```python
from build123d import *

# Parameters (mm, degrees)
SKETCH3_R          = 2.15
CUT_EXTRUDE1_DEPTH = 10
CHAMFER1_SIZE      = 0.4
CHAMFER2_SIZE      = 2
CHAMFER3_SIZE      = 2


with BuildPart() as part:
    # Sketch1 → Loft1 section 0
    with BuildSketch(Plane.XY):
        with BuildLine():
            Line((0, 0), (54, 0))
            Line((54, 0), (54, 10))
            Line((54, 10), (0, 10))
            Line((0, 10), (0, 0))
        make_face()
    # Sketch2 → Loft1 section 1
    with BuildSketch(Plane.XY.offset(9)):
        with BuildLine():
            Line((0, 9.5), (54, 9.5))
            Line((54, 9.5), (54, 0.5))
            Line((54, 0.5), (0, 0.5))
            Line((0, 0.5), (0, 9.5))
        make_face()
    loft()

    # Sketch3 → Cut-Extrude1 (cut)
    with BuildSketch(Plane(origin=(0, 0, 0), x_dir=(-1, 0, 0), z_dir=(0, 0, -1))):
        with Locations((-49.5, 5)):
            Circle(SKETCH3_R)
        with Locations((-4.5, 5)):
            Circle(SKETCH3_R)
    extrude(amount=-CUT_EXTRUDE1_DEPTH, mode=Mode.SUBTRACT)

    # Chamfer1
    chamfer1_edges = [part.edges().sort_by_distance(p)[0] for p in [
        (51.65, 5, 9),
        (51.65, 5, 0),
        (6.65, 5, 9),
        (6.65, 5, 0),
    ]]
    chamfer(chamfer1_edges, length=CHAMFER1_SIZE)

    # Chamfer2
    chamfer2_edges = [part.edges().sort_by_distance(p)[0] for p in [
        (0, 9.75, 4.5),
        (54, 9.75, 4.5),
    ]]
    chamfer(chamfer2_edges, length=CHAMFER2_SIZE)

    # Chamfer3
    chamfer3_edges = [part.edges().sort_by_distance(p)[0] for p in [
        (54, 0.25, 4.5),
        (0, 0.25, 4.5),
    ]]
    chamfer(chamfer3_edges, length=CHAMFER3_SIZE)


solid = part.part
```
The listing builds one solid part. Answer for the finished solid, in the listing's coordinates (mm). Give positions to 0.01 mm unless a question says otherwise; leave off trailing zeros. Loops run counter-clockwise (first coordinate to the right, second up) from the corner with the lowest first, then second, coordinate; pieces in that order, holes last. Notation, with made-up numbers: M 22,-20.75 L 69,-20.75 A38 ccw 69,18.25 Z; hole C 36,27 d9. An arc over 180 degrees is marked long. One line per item, written item: value.
Q1. A cutting plane is placed at C-C on x = 36. Determine the outline of the cut face in (y, z), then the cut area to 3 significant figures.
Working result:
outline: M 0,0 L 10,0 L 9.5,9 L 0.5,9 Z
area: 85.5 mm^2
Q2. A cutting plane is placed at A-A on x = 49.5. Determine the outline of the cut face in (y, z).
Working result:
outline: M 0,0 L 2.45,0 L 2.85,0.4 L 2.85,8.6 L 2.45,9 L 0.5,9 Z; M 7.15,0.4 L 7.55,0 L 10,0 L 9.5,9 L 7.55,9 L 7.15,8.6 Z
Q3. Determine the mould class of faces 1 (the face through (26.65, 0.253, 4.563)), 2 (the face through (47.45, 5.65, 4.44)), 3 (the face through (27, 5, 9)) for opening direction Y: +Y half, -Y half, draft (parallel to the pull), parting line (faces both ways), or undercut.
Working result:
face 1: -Y half
face 2: undercut
face 3: draft
Q4. A cutting plane is placed at B-B on y = 5. Give the number of separate pieces and of enclosed holes in the cut face, then the cut area to 3 significant figures.
Working result:
separate pieces: 3
enclosed holes: 0
area: 408 mm^2
Q5. Find the intervals of material crossed by line 1 (X direction, y = 4, z = 8.75); line 2 (X direction, y = 3.5, z = 8.75); line 3 (Y direction, x = 4.5, z = 5), in increasing order. Write a range as from..to.
Working result:
line 1: x = 0..2.43, 6.57..47.43, 51.57..54
line 2: x = 0..2.76, 6.24..47.76, 51.24..54
line 3: y = 0.28..2.85, 7.15..9.72
